Check sheet for the modelled part. Datum: model origin and axes. Units: mm. Face numbers are marked on the shaded views. Give positions to 0.01 mm unless a question says otherwise; leave off trailing zeros. Write each loop counter-clockwise with the first axis right and the second up, starting at its lowest first coordinate (ties: lowest second). Pieces come first, ordered by that corner, then holes.
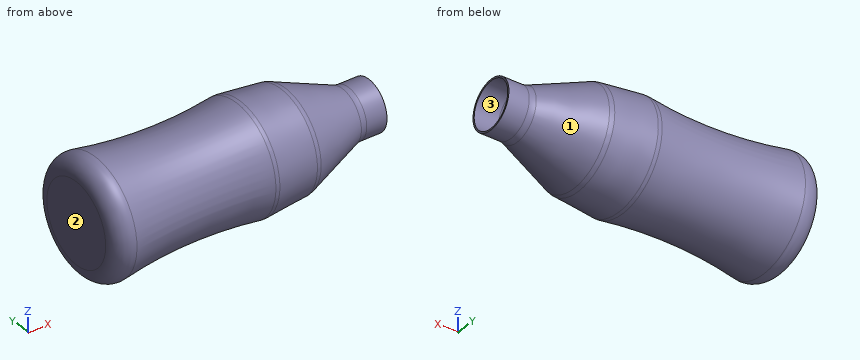
from build123d import *

# Parameters (mm, degrees)
FILLET1_R = 10


with BuildPart() as part:
    # Sketch1 → Revolve2 (revolve)
    with BuildSketch(Plane.XY, mode=Mode.PRIVATE) as revolve2_sk:
        with BuildLine():
            Line((-72.007624159, 0), (-72.007624159, 24.57))
            ThreePointArc((-72.007624159, 24.57), (-68.418740423, 32.244476415), (-60.228106509, 34.410392113))
            ThreePointArc((-60.228106509, 34.410392113), (-17.104532656, 30.124451731), (26.151893491, 32.75))
            Line((26.151893491, 32.75), (53.241893491, 30))
            Line((53.241893491, 30), (90.631893491, 15))
            Line((90.631893491, 15), (104.821893491, 15))
            Line((104.821893491, 15), (104.821893491, 14))
            Line((104.821893491, 14), (103.821893491, 14))
            Line((103.821893491, 14), (90.438785202, 14))
            Line((90.438785202, 14), (53.000518344, 29.019363543))
            Line((53.000518344, 29.019363543), (26.17157318, 31.74286296))
            ThreePointArc((26.17157318, 31.74286296), (-17.184498372, 29.125810874), (-60.406058274, 33.426352902))
            ThreePointArc((-60.406058274, 33.426352902), (-67.777628796, 31.477028774), (-71.007624159, 24.57))
            Line((-71.007624159, 24.57), (-71.007624159, 0))
            Line((-71.007624159, 0), (-72.007624159, 0))
        make_face()
    revolve(revolve2_sk.sketch.rotate(Axis((0, 0, 0), (-1, 0, 0)), 90), axis=Axis((0, 0, 0), (-1, 0, 0)))

    # Fillet1
    fillet1_edges = [part.edges().sort_by_distance(p)[0] for p in [
        (53.241893491, 0, 30),
        (90.631893491, 0, 15),
        (26.151893491, 0, 32.75),
    ]]
    fillet(fillet1_edges, radius=FILLET1_R)


solid = part.part
1) Sectioned sample at A-A on x = 49.5. Record the boundary of the cut face in (y, z).
2) Scan lines: L1, parallel to Y at x = 101.5, z = 0; L2, parallel to X at y = 12, z = 7; L3, parallel to Z at x = 55.5, y = 16. Record each from-to range of solid material in increasing order.
3) Draft check along Y on the marked faces 1, 2 and 3. Enter one of: +Y half, -Y half, draft (parallel to the pull), parting line (faces both ways), or undercut.
4) Sectioned sample at B-B on x = 19.5. Record the boundary of the cut face in (y, z).
5) Gauge pin test, flat ends, axial feed: pin 1 (6 mm diameter, centred on x = 75.5, z = 8.5, fed in from +Y); pin 2 (8 mm diameter, centred on x = -14.5, y = -23.5, fed in from +Z); pin 3 (10 mm diameter, centred on x = 9, z = 25.5, fed in from -Y); pin 4 (24.5 mm diameter, centred on y = 8.5, z = -10.5, fed in from +X). Record the tip position at first contact, or that the pin passes through.
Answers below:
1. outline: circle Ø60.76 at (0, 0); hole circle Ø58.75 at (0, 0)
2. L1: y = -15 to -14, 14 to 15
2. L2: x = -72.01 to -71.01
2. L3: z = -24.3 to -23, 23 to 24.3
3. face 1: parting line
3. face 2: draft
3. face 3: undercut
4. outline: circle Ø63.79 at (0, 0); hole circle Ø61.77 at (0, 0)
5. pin 1: stops at y = 20.99
5. pin 2: stops at z = 22.91
5. pin 3: stops at y = -23.12
5. pin 4: stops at x = 104.82
